Autodesk Inventor part; units mm, degrees
ref_plane "YZ Plane" through (0, 0, 0) normal (1, 0, 0) x (0, 1, 0)
ref_plane "XZ Plane" through (0, 0, 0) normal (0, 1, 0) x (-1, 0, 0)
ref_plane "XY Plane" through (0, 0, 0) normal (0, 0, 1) x (1, 0, 0)
sketch "Sketch1" plane through (0, 0, 0) normal (0, 0, 1) x (1, 0, 0)
  line L0 (-102.5157, 69.2842) -> (97.4843, 69.2842)
  line L1 (97.4843, 69.2842) -> (97.4843, -80.7158)
  line L2 (97.4843, -80.7158) -> (-102.5157, -80.7158)
  line L3 (-102.5157, -80.7158) -> (-102.5157, 69.2842)
  point P0 (0, 0)
extrude "Extrusion1" add sketch "Sketch1" along normal blind 3
sketch "Sketch3" plane through (0, 0, 3) normal (0, 0, 1) x (1, 0, 0)
  point P0 (0, 0)
sketch "Sketch4" plane through (0, 0, 3) normal (0, 0, 1) x (1, 0, 0)
  line L0 (97.4843, 69.2842) -> (-102.5157, 69.2842)
  line L1 (-102.5157, 69.2842) -> (-99.5157, 69.2842)
  line L2 (-99.5157, 69.2842) -> (-99.5157, 19.2842)
  line L3 (-99.5157, 19.2842) -> (-102.5157, 19.2842)
  line L4 (-102.5157, 19.2842) -> (-102.5157, 69.2842)
  point P0 (0, 0)
extrude "Extrusion2" cut sketch "Sketch4" against normal blind 3
sketch "Sketch5" plane through (0, 0, 3) normal (0, 0, 1) x (1, 0, 0)
  line L0 (97.4843, -80.7158) -> (94.4843, -80.7158)
  line L1 (94.4843, -80.7158) -> (94.4843, -30.7158)
  line L2 (94.4843, -30.7158) -> (97.4843, -30.7158)
  line L3 (97.4843, -30.7158) -> (97.4843, -80.7158)
  point P0 (0, 0)
  point P1 (-102.5157, -80.7158)
  dimension "d17" = 3
  dimension "d18" = 50
extrude "Extrusion3" cut sketch "Sketch5" against normal blind 3
sketch "Sketch6" plane through (0, 0, 3) normal (0, 0, 1) x (1, 0, 0)
  line L0 (97.4843, -30.7158) -> (97.4843, 69.2842)
  line L1 (97.4843, 69.2842) -> (94.4843, 69.2842)
  line L2 (94.4843, 69.2842) -> (94.4843, 19.2842)
  line L3 (94.4843, 19.2842) -> (97.4843, 19.2842)
  line L4 (97.4843, 19.2842) -> (97.4843, 69.2842)
  point P0 (0, 0)
  dimension "d21" = 50
  dimension "d22" = 3
extrude "Extrusion4" cut sketch "Sketch6" against normal blind 3
sketch "Sketch7" plane through (0, 0, 3) normal (0, 0, 1) x (1, 0, 0)
  line L0 (-102.5157, 19.2842) -> (-102.5157, -80.7158)
  line L1 (-102.5157, -80.7158) -> (-99.5157, -80.7158)
  line L2 (-99.5157, -80.7158) -> (-99.5157, -30.7158)
  line L3 (-99.5157, -30.7158) -> (-102.5157, -30.7158)
  line L4 (-102.5157, -30.7158) -> (-102.5157, -80.7158)
  point P0 (0, 0)
  dimension "d25" = 50
  dimension "d26" = 3
extrude "Extrusion5" cut sketch "Sketch7" against normal blind 3
sketch "Sketch8" plane through (0, 0, 3) normal (0, 0, 1) x (1, 0, 0)
  line L0 (-102.5157, -30.7158) -> (-102.5157, 19.2842)
  line L1 (97.4843, -30.7158) -> (94.4843, -30.7158)
  line L2 (94.4843, -80.7158) -> (-99.5157, -80.7158)
  line L3 (-10.0157, -50.7158) -> (4.9843, -50.7158)
  line L4 (4.9843, -50.7158) -> (4.9843, -80.7158)
  line L5 (4.9843, -80.7158) -> (-10.0157, -80.7158)
  line L6 (-10.0157, -80.7158) -> (-10.0157, -50.7158)
  point P0 (0, 0)
  dimension "d32" = 15
  dimension "d33" = 30
extrude "Extrusion6" cut sketch "Sketch8" against normal blind 3
sketch "Sketch9" plane through (-10.0157, -80.7158, 3) normal (1, 0, 0) x (0, 0, -1)
  point P0 (3, 80.7158)
sketch "Sketch10" plane through (-10.0157, -50.7158, 3) normal (0, -1, 0) x (1, 0, 0)
  line L0 (15, 0) -> (15, -3)
  line L1 (15, -3) -> (0, -3)
  line L2 (15, 0) -> (0, 0)
  line L3 (0, 0) -> (0, -3)
  line L4 (0, -3) -> (15, -3)
  line L5 (15, -3) -> (15, 0)
  point P0 (10.0157, -3)
extrude "Extrusion7" add sketch "Sketch10" along normal blind 30
sketch "Sketch11" plane through (0, 0, 3) normal (0, 0, 1) x (1, 0, 0)
  line L0 (94.4843, -80.7158) -> (-99.5157, -80.7158)
  line L1 (-99.5157, -80.7158) -> (-99.5157, -30.7158)
  line L2 (97.4843, 19.2842) -> (97.4843, -30.7158)
  line L3 (-102.5157, -30.7158) -> (-102.5157, 19.2842)
  line L4 (-99.5157, 69.2842) -> (94.4843, 69.2842)
  point P0 (0, 0)
sketch "Sketch12" plane through (0, 0, 3) normal (0, 0, 1) x (1, 0, 0)
  circle A0 centre (34.4088, 18.4314) radius 1.5
  circle A1 centre (33.1388, -29.8286) radius 1.5
  circle A2 centre (-41.7912, -29.8286) radius 1.5
  circle A3 centre (-48.1412, 18.4314) radius 1.5
  point P0 (0, 0)
extrude "Extrusion8" cut sketch "Sketch12" against normal blind 3
sketch "Sketch13" plane through (0, 0, 3) normal (0, 0, 1) x (1, 0, 0)
  line L0 (-99.5157, 69.2842) -> (94.4843, 69.2842)
  line L1 (-102.5157, -30.7158) -> (-102.5157, 19.2842)
  line L2 (94.4843, -80.7158) -> (-99.5157, -80.7158)
  line L3 (-85.4157, 20.4542) -> (-70.4157, 20.4542)
  line L4 (-70.4157, 20.4542) -> (-70.4157, -31.8858)
  line L5 (-70.4157, -31.8858) -> (-85.4157, -31.8858)
  line L6 (-85.4157, -31.8858) -> (-85.4157, 20.4542)
  line L7 (-53.3157, 45.7842) -> (48.2843, 45.7842)
  line L8 (48.2843, 45.7842) -> (48.2843, 60.7842)
  line L9 (48.2843, 60.7842) -> (-53.3157, 60.7842)
  line L10 (-53.3157, 60.7842) -> (-53.3157, 45.7842)
  line L11 (65.3843, 20.4542) -> (80.3843, 20.4542)
  line L12 (80.3843, 20.4542) -> (80.3843, -31.8858)
  line L13 (80.3843, -31.8858) -> (65.3843, -31.8858)
  line L14 (65.3843, -31.8858) -> (65.3843, 20.4542)
  line L15 (97.4843, -30.7158) -> (97.4843, 19.2842)
  line L16 (94.4843, 69.2842) -> (94.4843, 19.2842)
  line L17 (-99.5157, 19.2842) -> (-99.5157, 69.2842)
  line L18 (-53.3157, -72.2158) -> (48.2843, -72.2158)
  line L19 (48.2843, -72.2158) -> (48.2843, -57.2158)
  line L20 (48.2843, -57.2158) -> (-53.3157, -57.2158)
  line L21 (-53.3157, -57.2158) -> (-53.3157, -72.2158)
  line L22 (-99.5157, -30.7158) -> (-99.5157, -80.7158)
  line L23 (94.4843, -30.7158) -> (94.4843, -80.7158)
  point P0 (0, 0)
extrude "Extrusion9" cut sketch "Sketch13" against normal blind 3
sketch "Sketch14" plane through (0, 0, 3) normal (0, 0, 1) x (1, 0, 0)
  point P0 (0, 0)
properties part number "Level3"
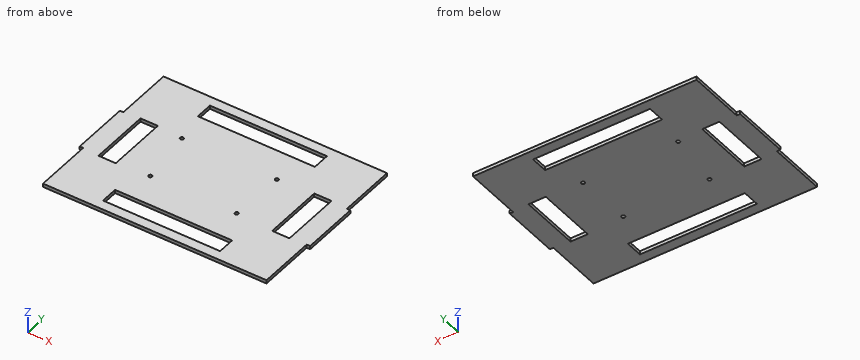
The listing builds one solid part. Answer for the finished solid, in the listing's coordinates (mm). Round coordinates to 2 decimals unless told otherwise and drop trailing zeros. Write each loop counter-clockwise with the first axis right and the second up, starting at its lowest first coordinate (ties: lowest second). Pieces come first, ordered by that corner, then holes. Notation, with made-up numbers: (86, 7.5) -> (90, 7.5) arc R8 cw to (90, 22.5) -> close; hole circle Ø7 at (82.25, 25.5). An arc over 180 degrees is marked (long way). Use CSV: the item, a comma, the result in double quotes. Start each with the question number.
(1) Section A-A on y = -20 is taken. Give the vertices of the cut face in (x, z), then the cut area to 3 significant figures.
(2) Section B-B on x = -83 is taken. Give the vertices of the cut face in (y, z).
(3) Section C-C on x = -29.5 is taken. Give the vertices of the cut face in (y, z), then the cut area to 3 significant figures.
(4) Each of these flat-tipped pins is pushed along its axis until it touches: pin 1 (0.9 mm diameter, centred on y = 51, z = 2, fed in from +X); pin 2 (2.5 mm diameter, centred on x = 34.41, y = 18.43, fed in from +Z); pin 3 (1.5 mm diameter, centred on y = -67.5, z = 1, fed in from -X). Where does it stop, or does it pass through?
(5) Section D-D on y = -60.5 is taken. Give the vertices of the cut face in (x, z).
(6) Consider L1, parallel to Y at x = 45, z = 2.4; L2, parallel to X at y = -3.5, z = 1; L3, parallel to X at y = 53, z = 1.8. Determine where each line is inside the solid, lowest interval first. Write a range as from..to.
A:
1,outline,"(-102.52, 0) -> (-85.42, 0) -> (-85.42, 3) -> (-102.52, 3) -> close; (-70.42, 0) -> (65.38, 0) -> (65.38, 3) -> (-70.42, 3) -> close; (80.38, 0) -> (97.48, 0) -> (97.48, 3) -> (80.38, 3) -> close"
1,area,"510 mm²"
2,outline,"(-80.72, 0) -> (-31.89, 0) -> (-31.89, 3) -> (-80.72, 3) -> close; (20.45, 0) -> (69.28, 0) -> (69.28, 3) -> (20.45, 3) -> close"
3,outline,"(-80.72, 0) -> (-72.22, 0) -> (-72.22, 3) -> (-80.72, 3) -> close; (-57.22, 0) -> (45.78, 0) -> (45.78, 3) -> (-57.22, 3) -> close; (60.78, 0) -> (69.28, 0) -> (69.28, 3) -> (60.78, 3) -> close"
3,area,"360 mm²"
4,pin 1,"stops at x = 94.48"
4,pin 2,"passes through"
4,pin 3,"stops at x = -99.52"
5,outline,"(-99.52, 0) -> (-53.32, 0) -> (-53.32, 3) -> (-99.52, 3) -> close; (48.28, 0) -> (94.48, 0) -> (94.48, 3) -> (48.28, 3) -> close"
6,L1,"y = -80.72..-72.22, -57.22..45.78, 60.78..69.28"
6,L2,"x = -102.52..-85.42, -70.42..65.38, 80.38..97.48"
6,L3,"x = -99.52..-53.32, 48.28..94.48"
